from build123d import *

# Parameters (mm, degrees)
SKETCH024_R          = 5.03
PAD018_DEPTH         = 5
PAD019_DEPTH         = 22
SKETCH027_R          = 1.4
POCKET004_DEPTH      = 0.001
POCKET004_DEPTH_BACK = 22.001


with BuildPart() as part:
    # Sketch024 → Pad018 (new body)
    with BuildSketch(Plane.XY.offset(6)):
        Circle(SKETCH024_R)
    extrude(amount=PAD018_DEPTH)

    # Sketch025 → Pad019 (join)
    with BuildSketch(Plane.XY):
        Polygon((2.47, -4.278165), (4.94, 0), (2.47, 4.278165), (-2.47, 4.278165), (-4.94, 0), (-2.47, -4.278165), align=None)
    extrude(amount=PAD019_DEPTH)

    # Sketch026 → Revolution006 (revolve)
    with BuildSketch(Plane.XZ):
        Polygon((-5.03, 11), (-3.83, 11), (-3.83, 12.2), align=None)
        Polygon((-5.03, 6), (-3.83, 6), (-3.83, 4.8), align=None)
    revolve(axis=Axis((0, 0, 0), (0, 0, 1)))

    # Sketch027 → Pocket004 (cut, two sides)
    with BuildSketch(Plane.XY) as pocket004_sk:
        Circle(SKETCH027_R)
    extrude(amount=-POCKET004_DEPTH, mode=Mode.SUBTRACT)
    extrude(pocket004_sk.sketch, amount=POCKET004_DEPTH_BACK, mode=Mode.SUBTRACT)


solid = part.part
Source: CAD feature listing. Evaluate the final solid. Frame: model axes, mm. A direction names the side the tool comes from. Coordinates: 2 decimals unless noted, no trailing zeros. Loops run counter-clockwise (first coordinate to the right, second up) from the corner with the lowest first, then second, coordinate; pieces in that order, holes last. Notation, with made-up numbers: (21.5, 81.25) - (66.5, 81.25) arc R13 cw to (66.5, 102.25) - close; hole circle Ø3 at (-21.5, 34). An arc over 180 degrees is marked (long way). One line per question, with ' | ' between items.
1) Set-up query: faces 1 (the face through (3.72, 2.11, 2.91)), 2 (the face through (3.72, 2.11, 16.47)), 3 (the face through (-3.688, 2.169, 16.469)). Return all of +Z, -Z, +X, -X, +Y, -Y with unobstructed straight access to the full face (end or side cutting, diameter ignored); none if empty.
Report:
face 1: -Z, +X, +Y | face 2: +Z, +X, +Y | face 3: +Z, -X, +Y
2) Line query: line 1 along Y through (x, z) = (0, 16); line 2 along X through (y, z) = (0, 8). Output: solid intervals per line, ascending.
Report:
line 1: y = -4.28 to -1.4, 1.4 to 4.28 | line 2: x = -5.03 to -1.4, 1.4 to 5.03
3) Section B-B, the plane x = 0. Return loops of the section in (y, z), then the cut area to 3 significant figures.
Report:
outline: (-5.03, 6) - (-4.28, 5.25) - (-4.28, 0) - (-1.4, 0) - (-1.4, 22) - (-4.28, 22) - (-4.28, 11.75) - (-5.03, 11) - close; (1.4, 0) - (4.28, 0) - (4.28, 5.25) - (5.03, 6) - (5.03, 11) - (4.28, 11.75) - (4.28, 22) - (1.4, 22) - close | area: 135 mm²
4) Section A-A, the plane z = 2.5. Return loops of the section in (x, y).
Report:
outline: (-4.94, 0) - (-2.47, -4.28) - (2.47, -4.28) - (4.94, 0) - (2.47, 4.28) - (-2.47, 4.28) - close; hole circle Ø2.8 at (0, 0)
5) First-contact query: P1, Ø1.5, axis at y = 3, z = 19, coming from the -X side; P2, Ø1.7, axis at x = 0, y = 0, coming from the -Z side; P3, Ø5.5, axis at x = -0.5, z = 3, coming from the -Y side; P4, Ø2.5, axis at x = -0.5, z = 17, coming from the -Y side. Flat tips, straight axial feed; report the tip coordinate or a pass-through.
Report:
P1: stops at x = -3.64 | P2: passes through | P3: stops at y = -4.76 | P4: stops at y = -4.28
6) Pull-direction query (Y, two-part tool) for faces 4 (the face through (-1.4, 0.06, 10.85)), 5 (the face through (3.688, -2.169, 2.914)), 6 (the face through (-3.688, 2.169, 2.914)); classes: released by +Y, released by -Y, zero draft, split by the parting line, or undercut.
Report:
face 4: undercut | face 5: released by -Y | face 6: released by +Y
7) Section C-C, the plane z = 8. Return loops of the section in (x, y).
Report:
outline: circle Ø10.06 at (0, 0); hole circle Ø2.8 at (0, 0)
